The model under review builds one solid part; all positions refer to its coordinate system, in mm. Give positions to 0.01 mm unless a question says otherwise; leave off trailing zeros. Loops run counter-clockwise (first coordinate to the right, second up) from the corner with the lowest first, then second, coordinate; pieces in that order, holes last. Notation, with made-up numbers: (69.5, -25.5) - (98.5, -25.5) arc R12 cw to (98.5, -8.5) - close; hole circle Ø7 at (-19, 44). An arc over 180 degrees is marked (long way). Answer as a JSON object with one key per item and string values.
from build123d import *

# Parameters (mm, degrees)
SKETCH1_R           = 35
SKETCH1_R_2         = 10.3
BOSS_EXTRUDE1_DEPTH = 6
SKETCH3_R           = 1.7
CUT_EXTRUDE1_DEPTH  = 50.859803449
SKETCH5_R           = 2.25
CUT_EXTRUDE2_DEPTH  = 50.859803449


with BuildPart() as part:
    # Sketch1 → Boss-Extrude1 (new body)
    with BuildSketch(Plane(origin=(0, 0, 0), x_dir=(1, 0, 0), z_dir=(0, 1, 0))):
        with Locations(Location((0, 0, 0), (0, 0, 270))):
            Circle(SKETCH1_R)
        with Locations(Location((0, 0, 0), (0, 0, 270))):
            Circle(SKETCH1_R_2, mode=Mode.SUBTRACT)
    extrude(amount=BOSS_EXTRUDE1_DEPTH)

    # Sketch3 → Cut-Extrude1 (cut, through all)
    with BuildSketch(Plane(origin=(0, 6, 0), x_dir=(1, 0, 0), z_dir=(0, 1, 0))):
        with Locations(Location((-20.8, 0, 0), (0, 0, 270))):
            Circle(SKETCH3_R)
        with Locations(Location((0, 20.8, 0), (0, 0, 270))):
            Circle(SKETCH3_R)
        with Locations(Location((20.8, 0, 0), (0, 0, 270))):
            Circle(SKETCH3_R)
        with Locations(Location((0, -20.8, 0), (0, 0, 270))):
            Circle(SKETCH3_R)
    extrude(amount=-CUT_EXTRUDE1_DEPTH, mode=Mode.SUBTRACT)

    # Sketch5 → Cut-Extrude2 (cut, through all)
    with BuildSketch(Plane(origin=(0, 6, 0), x_dir=(1, 0, 0), z_dir=(0, 1, 0))):
        with Locations(Location((-20.506096654, 20.506096654, 0), (0, 0, 270))):
            Circle(SKETCH5_R)
        with Locations(Location((-20.506096654, -20.506096654, 0), (0, 0, 270))):
            Circle(SKETCH5_R)
        with Locations(Location((20.506096654, 20.506096654, 0), (0, 0, 270))):
            Circle(SKETCH5_R)
        with Locations(Location((20.506096654, -20.506096654, 0), (0, 0, 270))):
            Circle(SKETCH5_R)
    extrude(amount=-CUT_EXTRUDE2_DEPTH, mode=Mode.SUBTRACT)


solid = part.part
Q1. Consider section C-C, the plane z = 8.5. State the section outline as (x, y) points, plus the area to 3 significant figures.
Results:
{"outline": "(-33.95, 0) - (-5.82, 0) - (-5.82, 6) - (-33.95, 6) - close; (5.82, 0) - (33.95, 0) - (33.95, 6) - (5.82, 6) - close", "area": "338 mm^2"}
Q2. Consider section B-B, the plane x = -3. State the section outline as (y, z) points.
Results:
{"outline": "(0, -34.87) - (6, -34.87) - (6, -9.85) - (0, -9.85) - close; (0, 9.85) - (6, 9.85) - (6, 34.87) - (0, 34.87) - close"}
Q3. Consider section D-D, the plane y = 4.4. State how many separate pieces and enclosed holes the cut face has, plus the area to 3 significant figures.
Results:
{"separate pieces": "1", "enclosed holes": "9", "area": "3,420 mm^2"}
Q4. The part is to be moulded in two halves that separate along X. For faces 1 (the face through (-21, 3, -28)), 2 (the face through (22.486, 3.042, -0.221)), 3 (the face through (-7, 0, -8)), say which applies: +X half, -X half, draft (parallel to the pull), parting line (faces both ways), or undercut.
Results:
{"face 1": "parting line", "face 2": "undercut", "face 3": "draft"}
Q5. Clearance check with flat-ended pins moving along their axes: pin 1 Ø5 at (x, z) = (20.51, 20.51) entering from -Y; pin 2 Ø2 at (y, z) = (1.5, -6.5) entering from +X; pin 3 Ø2.5 at (x, z) = (0, 20.8) entering from +Y. State where each tip first meets the part, or that it passes through.
Results:
{"pin 1": "stops at y = 0", "pin 2": "stops at x = 34.57", "pin 3": "passes through"}
Q6. To check wall thickness, follow probe 1 along Z at (x, y) = (22, 3.3); probe 2 along X at (y, z) = (2.15, 20.8); probe 3 along X at (y, z) = (1.9, -1.5). State the ranges of each line that lie inside material, in increasing order. Write a range as [from, to].
Results:
{"probe 1": "z = [-27.22, -22.19], [-18.82, -1.2], [1.2, 18.82], [22.19, 27.22]", "probe 2": "x = [-28.15, -22.74], [-18.28, -1.7], [1.7, 18.28], [22.74, 28.15]", "probe 3": "x = [-34.97, -21.6], [-20, -10.19], [10.19, 20], [21.6, 34.97]"}
Q7. Consider section A-A, the plane z = 0. State the section outline as (x, y) points, plus the area to 3 significant figures.
Results:
{"outline": "(-35, 0) - (-22.5, 0) - (-22.5, 6) - (-35, 6) - close; (-19.1, 0) - (-10.3, 0) - (-10.3, 6) - (-19.1, 6) - close; (10.3, 0) - (19.1, 0) - (19.1, 6) - (10.3, 6) - close; (22.5, 0) - (35, 0) - (35, 6) - (22.5, 6) - close", "area": "256 mm^2"}
